from build123d import *

# Parameters (mm, degrees)
AUFSATZ_LINEAR_AUSTRAGEN1_DEPTH      = 120
F_3_4_3_4_DURCHMESSER_BOHRUNG1_D     = 3.4
F_3_4_3_4_DURCHMESSER_BOHRUNG1_DEPTH = 5
F_3_4_3_4_DURCHMESSER_BOHRUNG1_TIP   = 1.021463052


with BuildPart() as part:
    # Skizze1 → Aufsatz-Linear austragen1 (new body)
    with BuildSketch(Plane.XY):
        with BuildLine():
            Line((0, 0), (15, 0))
            Line((15, 0), (15, 3))
            ThreePointArc((15, 3), (32, 20), (49, 3))
            Line((49, 3), (49, 0))
            Line((49, 0), (64, 0))
            Line((64, 0), (64, 3))
            Line((64, 3), (52, 3))
            ThreePointArc((52, 3), (32, 23), (12, 3))
            Line((12, 3), (0, 3))
            Line((0, 3), (0, 0))
        make_face()
    extrude(amount=AUFSATZ_LINEAR_AUSTRAGEN1_DEPTH)

    # Ø3.4 (3.4) Durchmesser Bohrung1
    with Locations(Plane(origin=(0, 3, 0), x_dir=(1, 0, 0), z_dir=(0, 1, 0))):
        with Locations((58, -60), (6, -60)):
            Hole(F_3_4_3_4_DURCHMESSER_BOHRUNG1_D / 2, depth=F_3_4_3_4_DURCHMESSER_BOHRUNG1_DEPTH)
            with Locations((0, 0, -(F_3_4_3_4_DURCHMESSER_BOHRUNG1_DEPTH + F_3_4_3_4_DURCHMESSER_BOHRUNG1_TIP / 2))):  # 118° drill point
                Cone(0, F_3_4_3_4_DURCHMESSER_BOHRUNG1_D / 2, F_3_4_3_4_DURCHMESSER_BOHRUNG1_TIP, mode=Mode.SUBTRACT)


solid = part.part
The model under review builds one solid part; all positions refer to its coordinate system, in mm. A direction names the side the tool comes from. Coordinates: 2 decimals unless noted, no trailing zeros. Loops run counter-clockwise (first coordinate to the right, second up) from the corner with the lowest first, then second, coordinate; pieces in that order, holes last. Notation, with made-up numbers: M 77,53 L 118,53 A32 cw 118,91 Z; hole C 73,22 d11. An arc over 180 degrees is marked long. Put each result on its own line as item: value. Start each with the question number.
Q1. For faces 1 (the flat face through (9, 3, 59)), 2 (the flat face through (15, 1, 59)), 3 (the flat face through (55, 3, 59)), 4 (the flat face through (64, 1, 59)), list the 3-axis set-ups (+Z, -Z, +X, -X, +Y, -Y) from which the entire face can be reached by the end or side of a thin tool; tool diameter is ignored.
Q2. The part is to be moulded in two halves that separate along Z. For faces 5 (the flat face through (0, 2, 59)), 6 (the flat face through (29, 20, 120)), 7 (the cylindrical face through (59.7, 1.48, 59.93)), 8 (the cylindrical face through (6.221, 1.479, 58.314)), say which applies: +Z half, -Z half, draft (parallel to the pull), parting line (faces both ways), or undercut.
Q3. Add section D-D (z = 90). Write out the cut boundary in (x, y).
Q4. Add section B-B (x = 6). Write out the cut boundary in (y, z).
Q5. Wall thickness on line 1 (X direction, y = 0.75, z = 60); line 2 (X direction, y = 3.25, z = 100); line 3 (Z direction, x = 58, y = 1.85): over which ranges is each line inside the solid? List them lowest first.
Q6. Clearance check with flat-ended pins moving along their axes: pin 1 (1 mm diameter, centred on y = 7.5, z = 52.5, fed in from -X); pin 2 (8 mm diameter, centred on y = 6.5, z = 37, fed in from +X); pin 3 (6 mm diameter, centred on x = 59.5, z = 34, fed in from +Y); pin 4 (9.5 mm diameter, centred on x = 9, z = 41, fed in from +Y). State where each tip first meets the part, or that it passes through.
Q7. Add section A-A (z = 60). Write out the cut boundary in (x, y).
Q8. Add section C-C (y = 16.5). Write out the cut boundary in (x, z), and give its area (3 significant figures).
Answers:
1. face 1: +Z, -Z, -X, +Y
1. face 2: +Z, -Z, -Y
1. face 3: +Z, -Z, +X, +Y
1. face 4: +Z, -Z, +X, +Y, -Y
2. face 5: draft
2. face 6: +Z half
2. face 7: undercut
2. face 8: undercut
3. outline: M 0,0 L 15,0 L 15,3 A17 cw 49,3 L 49,0 L 64,0 L 64,3 L 52,3 A20 ccw 12,3 L 0,3 Z
4. outline: M 0,0 L 3,0 L 3,58.3 L 0,58.3 Z; M 0,61.7 L 3,61.7 L 3,120 L 0,120 Z
5. line 1: x = 0 to 4.3, 7.7 to 15, 49 to 56.3, 59.7 to 64
5. line 2: x = 12 to 15, 49 to 52
5. line 3: z = 0 to 58.3, 61.7 to 120
6. pin 1: stops at x = 12.4
6. pin 2: stops at x = 64
6. pin 3: stops at y = 3
6. pin 4: stops at y = 11.18
7. outline: M 0,0 L 4.3,0 L 4.3,3 L 0,3 Z; M 7.7,0 L 15,0 L 15,3 A17 cw 49,3 L 49,0 L 56.3,0 L 56.3,3 L 52,3 A20 ccw 12,3 L 7.7,3 Z; M 59.7,0 L 64,0 L 64,3 L 59.7,3 Z
8. outline: M 17.24,0 L 21.67,0 L 21.67,120 L 17.24,120 Z; M 42.33,0 L 46.76,0 L 46.76,120 L 42.33,120 Z
8. area: 1,060 mm^2
